For this review, take the finished solid that the model builds, in its own axes (mm). A direction names the side the tool comes from. Round coordinates to 2 decimals unless told otherwise and drop trailing zeros. Write each loop counter-clockwise with the first axis right and the second up, starting at its lowest first coordinate (ties: lowest second). Pieces come first, ordered by that corner, then holes. Notation, with made-up numbers: (54.5, 3.25) -> (63.5, 3.25) arc R36 cw to (63.5, 41.25) -> close; hole circle Ø7 at (4.5, -7.75). An arc over 180 degrees is marked (long way). Answer in a Markdown table with one row per item. Add a question column.
```python
from build123d import *

# Parameters (mm, degrees)
SKETCH1_R           = 11
BOSS_EXTRUDE1_DEPTH = 9
SKETCH2_R           = 4
CUT_EXTRUDE1_DEPTH  = 10
SKETCH3_R           = 9
SKETCH3_R_2         = 6
CUT_EXTRUDE2_DEPTH  = 0.2
SKETCH4_R           = 9
SKETCH4_R_2         = 6
CUT_EXTRUDE3_DEPTH  = 0.2
SKETCH5_R           = 6
SKETCH5_R_2         = 4
BOSS_EXTRUDE2_DEPTH = 5


with BuildPart() as part:
    # Sketch1 → Boss-Extrude1 (new body)
    with BuildSketch(Plane.XY):
        Circle(SKETCH1_R)
    extrude(amount=BOSS_EXTRUDE1_DEPTH)

    # Sketch2 → Cut-Extrude1 (cut, through all)
    with BuildSketch(Plane.XY.offset(9)):
        Circle(SKETCH2_R)
    extrude(amount=-CUT_EXTRUDE1_DEPTH, mode=Mode.SUBTRACT)

    # Sketch3 → Cut-Extrude2 (cut)
    with BuildSketch(Plane.XY.offset(9)):
        Circle(SKETCH3_R)
        Circle(SKETCH3_R_2, mode=Mode.SUBTRACT)
    extrude(amount=-CUT_EXTRUDE2_DEPTH, mode=Mode.SUBTRACT)

    # Sketch4 → Cut-Extrude3 (cut)
    with BuildSketch(Plane(origin=(0, 0, 0), x_dir=(-1, 0, 0), z_dir=(0, 0, -1))):
        Circle(SKETCH4_R)
        Circle(SKETCH4_R_2, mode=Mode.SUBTRACT)
    extrude(amount=-CUT_EXTRUDE3_DEPTH, mode=Mode.SUBTRACT)

    # Sketch5 → Boss-Extrude2 (add)
    with BuildSketch(Plane.XY.offset(9)):
        Circle(SKETCH5_R)
        Circle(SKETCH5_R_2, mode=Mode.SUBTRACT)
    extrude(amount=BOSS_EXTRUDE2_DEPTH)


solid = part.part
```
1. We need section D-D (x = 7). Write out the cut boundary in (y, z).
2. We need section A-A (y = 0). Write out the cut boundary in (x, z).
3. For L1, parallel to Y at x = 0, z = 8.9; L2, parallel to Y at x = 0, z = 10.2; L3, parallel to Y at x = 0, z = 2, list the stretches that pass through material, from the lowest coordinate up. Write a range as [from, to].
4. Tool access review of faces 4 (the flat face through (2, -9, 9)), 5 (the flat face through (-2, -6, 0.2)), 6 (the flat face through (-1.42, -3.92, 14)): name each direction out of +Z, -Z, +X, -X, +Y, -Y from which nothing blocks a thin tool from reaching the whole face with its end or side.
5. Clearance check with flat-ended pins moving along their axes: pin 1 Ø4 at (x, z) = (6.5, 11.5) entering from -Y; pin 2 Ø5 at (x, y) = (0, 0) entering from +Z; pin 3 Ø5 at (x, z) = (8.5, 6.5) entering from +Y; pin 4 Ø6 at (x, z) = (-6.5, 4.5) entering from +Y. State where each tip first meets the part, or that it passes through.
6. We need section C-C (z = 12.5). Write out the cut boundary in (x, y).
7. The part is to be moulded in two halves that separate along Y. For faces 1 (the flat face through (2, -6, 8.8)), 2 (the cylindrical face through (-2.38, -10.74, 4.44)), 3 (the flat face through (-1.42, -3.92, 0)), say which applies: pulls with the +Y half, pulls with the -Y half, needs draft (parallel to the pull), parting line crosses it, or undercut.
Response:
| question | item | result |
|---|---|---|
| 1 | outline | (-8.49, 0) -> (-5.66, 0) -> (-5.66, 0.2) -> (5.66, 0.2) -> (5.66, 0) -> (8.49, 0) -> (8.49, 9) -> (5.66, 9) -> (5.66, 8.8) -> (-5.66, 8.8) -> (-5.66, 9) -> (-8.49, 9) -> close |
| 2 | outline | (-11, 0) -> (-9, 0) -> (-9, 0.2) -> (-6, 0.2) -> (-6, 0) -> (-4, 0) -> (-4, 14) -> (-6, 14) -> (-6, 8.8) -> (-9, 8.8) -> (-9, 9) -> (-11, 9) -> close; (4, 0) -> (6, 0) -> (6, 0.2) -> (9, 0.2) -> (9, 0) -> (11, 0) -> (11, 9) -> (9, 9) -> (9, 8.8) -> (6, 8.8) -> (6, 14) -> (4, 14) -> close |
| 3 | L1 | [-11, -9], [-6, -4], [4, 6], [9, 11] |
| 3 | L2 | [-6, -4], [4, 6] |
| 3 | L3 | [-11, -4], [4, 11] |
| 4 | face 4 | +Z |
| 4 | face 5 | -Z |
| 4 | face 6 | +Z, +X, -X, +Y, -Y |
| 5 | pin 1 | y = -3.97 |
| 5 | pin 2 | through |
| 5 | pin 3 | y = 9.22 |
| 5 | pin 4 | y = 10.43 |
| 6 | outline | circle Ø12 at (0, 0); hole circle Ø8 at (0, 0) |
| 7 | face 1 | undercut |
| 7 | face 2 | parting line crosses it |
| 7 | face 3 | needs draft |
